Could you check a few things on this model? Use its own coordinates, in mm. A direction names the side the tool comes from. Give positions to 0.01 mm unless a question says otherwise; leave off trailing zeros. Loops run counter-clockwise (first coordinate to the right, second up) from the corner with the lowest first, then second, coordinate; pieces in that order, holes last. Notation, with made-up numbers: M -20.75,-4.75 L 36.25,-4.75 A6 ccw 36.25,4.25 Z; hole C 28.25,76.5 d9. An arc over 180 degrees is marked long. Answer in a Markdown table with one row per item. Add a question column.
1. I need wall thicknesses on line 1 along Y through (x, z) = (46, -34.5); line 2 along X through (y, z) = (-5.25, -23.5); line 3 along Z through (x, y) = (11.5, -12.25). Which ranges of each line are inside material? Lowest first, please. Write a range as from..to.
2. I'm going to push flat-ended pins straight in: pin 1 Ø8.5 at (x, y) = (33.5, -8) entering from +Z; pin 2 Ø12 at (x, z) = (20, -52.5) entering from +Y. Where does each tip first touch, or does it pass through?
3. Thinking about a two-plate mould opening in Y: for faces 3 (the flat face through (25, -21.814, -30)), 4 (the flat face through (0, -11, -30)), 5 (the flat face through (25, -19.274, -29)), 6 (the flat face through (25, 0, -30)), which applies, released by +Y, released by -Y, zero draft, split by the parting line, or undercut?
4. If we section it at B-B on y = -12.75: List the corners of the cut face in (x, z) for me.
5. Which directions (+Z, -Z, +X, -X, +Y, -Y) give clear straight access to the entire face, cutting with the end or side of a thin tool? Please do faces 1 (the flat face through (25, -11, -61.214)), 2 (the flat face through (25, -11, -58.674)).
6. If we section it at C-C on x = 42: List the corners of the cut face in (y, z) for me, then the cut area to 3 significant figures.
7. If we section it at A-A on z = -3.5: List the corners of the cut face in (x, y) for me.
```python
from build123d import *

# Parameters (mm, degrees)
F0_W     = 50.382692
F0_H     = 21.813512
F1_DEPTH = 61.214
F2_T     = -2.54


with BuildPart() as f1:
    # F0 (on Top) → F1 (new body)
    with BuildSketch(Plane.XY):
        with Locations((25.191346, -10.906756)):
            Rectangle(F0_W, F0_H)
    extrude(amount=-F1_DEPTH)

    # F2
    f2_openings = [f1.faces().sort_by_distance(p)[0] for p in [
        (25.191346, -10.906756, 0),
    ]]
    offset(amount=F2_T, openings=f2_openings)


solid = f1.part
```
Results:
| question | item | result |
|---|---|---|
| 1 | line 1 | -21.81..-19.27, -2.54..0 |
| 1 | line 2 | 0..2.54, 47.84..50.38 |
| 1 | line 3 | -61.21..-58.67 |
| 2 | pin 1 | z = -58.67 |
| 2 | pin 2 | y = 0 |
| 3 | face 3 | released by -Y |
| 3 | face 4 | zero draft |
| 3 | face 5 | undercut |
| 3 | face 6 | released by +Y |
| 4 | outline | M 0,-61.21 L 50.38,-61.21 L 50.38,0 L 47.84,0 L 47.84,-58.67 L 2.54,-58.67 L 2.54,0 L 0,0 Z |
| 5 | face 1 | -Z, +X, -X, +Y, -Y |
| 5 | face 2 | +Z |
| 6 | outline | M -21.81,-61.21 L 0,-61.21 L 0,0 L -2.54,0 L -2.54,-58.67 L -19.27,-58.67 L -19.27,0 L -21.81,0 Z |
| 6 | area | 353 mm2 |
| 7 | outline | M 0,-21.81 L 50.38,-21.81 L 50.38,0 L 0,0 Z; hole M 2.54,-19.27 L 47.84,-19.27 L 47.84,-2.54 L 2.54,-2.54 Z |
